Check sheet for the drawn part. Datum: minimum x, y, z corner. Units: mm. Give positions to 0.01 mm unless a question says otherwise; leave off trailing zeros. Order: outer loops, then holes, each group sorted by start corner. A loop starts at its lowest first (then second) coordinate and runs counter-clockwise, first axis right, second up. Notation, with made-up numbers: (-13, -1.5) - (13, -1.5) arc R28 ccw to (13, 26.5) - close; hole circle Ø2 at (-36.75, 33.5). An arc over 180 degrees is marked (long way). Answer as a JSON object with one key per item and string values. Group by question number.
(1) Section check A-A (x = 700). Record the boundary of the cut face in (y, z), then the cut area to 3 significant figures.
(2) Section check C-C (y = 33). Record the boundary of the cut face in (x, z).
(3) Thickness scan on line 1 (X direction, y = 158.5, z = 276); line 2 (Y direction, x = 424, z = 196); line 3 (Y direction, x = 162.5, z = 74) (1 decimal). Record the ranges inside material, lowest first.
(4) Section check B-B (z = 196). Record the boundary of the cut face in (x, y).
(5) Section check D-D (y = 266.5). Record the boundary of the cut face in (x, z), then the cut area to 3 significant figures.
(6) Depth check by flat-ended pin: pin 1 Ø6 at (x, z) = (165, 229) entering from +Y; pin 2 Ø5 at (y, z) = (271.5, 94) entering from -X (1 decimal); pin 3 Ø5 at (y, z) = (299.5, 213) entering from -X. Enter the tip coordinate at first touch or a pass-through.
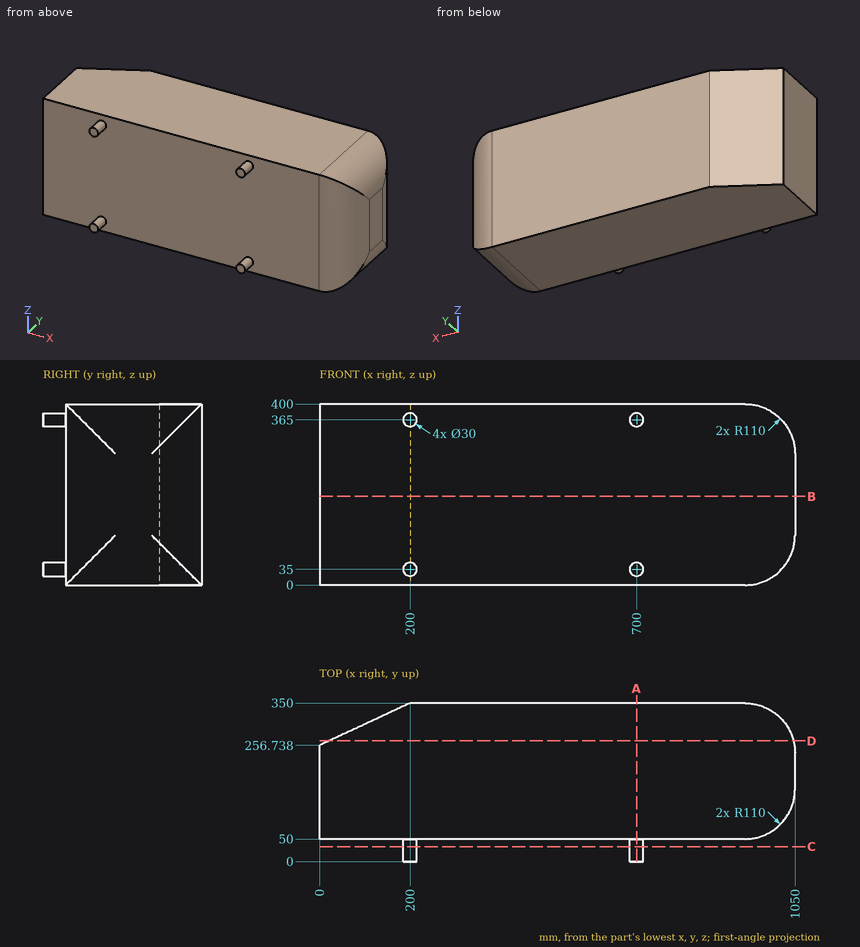
Solutions:
{
 "1": {"outline": "(0, 20) - (50, 20) - (50, 0) - (350, 0) - (350, 400) - (50, 400) - (50, 380) - (0, 380) - (0, 350) - (50, 350) - (50, 50) - (0, 50) - close", "area": "123,000 mm2"},
 "2": {"outline": "circle Ø30 at (200, 35); circle Ø30 at (200, 365); circle Ø30 at (700, 35); circle Ø30 at (700, 365)"},
 "3": {"line 1": "x = 0 to 1049.99", "line 2": "y = 50 to 350", "line 3": "y = 50 to 332.5"},
 "4": {"outline": "(0, 50) - (940, 50) arc R110 ccw to (1050, 160) - (1050, 240) arc R110 ccw to (940, 350) - (200, 350) - (0, 256.74) - close"},
 "5": {"outline": "(20.93, 0) - (940, 0) arc R110 ccw to (1046.76, 83.5) - (1046.76, 316.5) arc R110 ccw to (940, 400) - (20.93, 400) - close", "area": "406,000 mm2"},
 "6": {"pin 1": "stops at y = 335.08", "pin 2": "stops at x = 26.3", "pin 3": "stops at x = 86.34"}
}
